Verification items for the finished model (mm, model axes). A direction names the side the tool comes from. Coordinates: 2 decimals unless noted, no trailing zeros. Loops run counter-clockwise (first coordinate to the right, second up) from the corner with the lowest first, then second, coordinate; pieces in that order, holes last.
Q1. Mould release check, pull along Z, two halves, no side actions. Record for faces 3 (the face through (1, 1, 0)), 4 (the face through (2.54, 1, -1)), 5 (the face through (1, 0.381, -2)): +Z half, -Z half, draft (parallel to the pull), parting line (faces both ways), or undercut.
Q2. Go/stop test with flat-tipped pins: P1, Ø0.5, axis at y = -1.5, z = -1.5, coming from the -X side; P2, Ø0.7, axis at x = 1.5, y = 6.5, coming from the -Z side; P3, Ø0.7, axis at x = 1, y = -0.5, coming from the +Z side. Record where each tip stops, or that it passes through.
Q3. Access from +Z, -Z, +X, -X, +Y, -Y to the whole of each face (thin tool, end or side, straight path). Record for faces 1 (the face through (0.7, 2.54, -1.3)), 2 (the face through (0, 1, -1)).
Q4. Sectioned sample at A-A (x = 1.9). Enter the section's corners in (y, z), then the cut area to 3 significant figures.
Q5. Sectioned sample at B-B (y = 7.5). Enter the section's corners in (x, z), then the cut area to 3 significant figures.
Q6. Material ranges on probe 1 along Z at (x, y) = (1, 0.25); probe 2 along Y at (x, z) = (1.35, -0.45); probe 3 along Z at (x, y) = (1.5, 3.25), recorded low to high.
Q7. Sectioned sample at C-C (z = -2.35). Enter the section's corners in (x, y), then the cut area to 3 significant figures.
```python
from build123d import *

# Parameters (mm, degrees)
SKETCH1_W             = 2.54
SKETCH1_H             = 2.54
MAIN_BODY_DEPTH       = 2.54
SKETCH3_W             = 1.778
SKETCH3_H             = 0.381
CUT_EXTRUDE1_DEPTH    = 3.54
CUT_EXTRUDE2_DEPTH    = 3.54
SKETCH2_W             = 0.64
SKETCH2_H             = 0.64
PIN_DEPTH             = 6
PIN_DEPTH_BACK        = 5.54
CHAMFER1_SIZE         = 0.508
CHAMFER1_SIZE2        = 0.1905
CHAMFER1_PART_2_SIZE  = 0.508
CHAMFER1_PART_2_SIZE2 = 0.1905
CHAMFER1_PART_3_SIZE  = 0.508
CHAMFER1_PART_3_SIZE2 = 0.1905
CHAMFER1_PART_4_SIZE  = 0.508
CHAMFER1_PART_4_SIZE2 = 0.1905
CHAMFER2_SIZE         = 0.1905
CHAMFER2_SIZE2        = 0.508


with BuildPart() as part:
    # Sketch1 → Main Body (new body)
    with BuildSketch(Plane(origin=(0, 0, 0), x_dir=(1, 0, 0), z_dir=(0, 1, 0))):
        with Locations((1.27, 1.27)):
            Rectangle(SKETCH1_W, SKETCH1_H)
    extrude(amount=MAIN_BODY_DEPTH)

    # Sketch3 → Cut-Extrude1 (cut, through all)
    with BuildSketch(Plane.ZY):
        with Locations((-1.27, 0.1905)):
            Rectangle(SKETCH3_W, SKETCH3_H)
    extrude(amount=-CUT_EXTRUDE1_DEPTH, mode=Mode.SUBTRACT)

    # Sketch4 → Cut-Extrude2 (cut, through all)
    with BuildSketch(Plane(origin=(0, 2.54, 0), x_dir=(1, 0, 0), z_dir=(0, 1, 0))):
        Polygon((0.254, 2.54), (0, 2.54), (0, 2.032), align=None)
        Polygon((2.54, 2.54), (2.286, 2.54), (2.54, 2.032), align=None)
        Polygon((0.254, 0), (0, 0.508), (0, 0), align=None)
        Polygon((2.54, 0), (2.286, 0), (2.54, 0.508), align=None)
    extrude(amount=-CUT_EXTRUDE2_DEPTH, mode=Mode.SUBTRACT)

    # Sketch2 → Pin (add, two sides)
    with BuildSketch(Plane(origin=(0, 2.54, 0), x_dir=(1, 0, 0), z_dir=(0, 1, 0))) as pin_sk:
        with Locations((1.27, 1.27)):
            Rectangle(SKETCH2_W, SKETCH2_H)
    extrude(amount=PIN_DEPTH)
    extrude(pin_sk.sketch, amount=-PIN_DEPTH_BACK)

    # Chamfer1
    chamfer1_edges = [part.edges().sort_by_distance(p)[0] for p in [
        (0.95, 8.54, -1.27),
    ]]
    chamfer1_side = [part.faces().sort_by_distance(p)[0] for p in [
        (0.95, 5.54, -1.27),
    ]]
    chamfer(chamfer1_edges, length=CHAMFER1_SIZE, length2=CHAMFER1_SIZE2, reference=chamfer1_side[0])

    # Chamfer1 part 2
    chamfer1_part_2_edges = [part.edges().sort_by_distance(p)[0] for p in [
        (1.27, 8.54, -0.95),
    ]]
    chamfer1_part_2_side = [part.faces().sort_by_distance(p)[0] for p in [
        (1.27, 5.54, -0.95),
    ]]
    chamfer(chamfer1_part_2_edges, length=CHAMFER1_PART_2_SIZE, length2=CHAMFER1_PART_2_SIZE2, reference=chamfer1_part_2_side[0])

    # Chamfer1 part 3
    chamfer1_part_3_edges = [part.edges().sort_by_distance(p)[0] for p in [
        (1.59, 8.54, -1.27),
    ]]
    chamfer1_part_3_side = [part.faces().sort_by_distance(p)[0] for p in [
        (1.59, 5.54, -1.27),
    ]]
    chamfer(chamfer1_part_3_edges, length=CHAMFER1_PART_3_SIZE, length2=CHAMFER1_PART_3_SIZE2, reference=chamfer1_part_3_side[0])

    # Chamfer1 part 4
    chamfer1_part_4_edges = [part.edges().sort_by_distance(p)[0] for p in [
        (1.27, 8.54, -1.59),
    ]]
    chamfer1_part_4_side = [part.faces().sort_by_distance(p)[0] for p in [
        (1.27, 5.54, -1.59),
    ]]
    chamfer(chamfer1_part_4_edges, length=CHAMFER1_PART_4_SIZE, length2=CHAMFER1_PART_4_SIZE2, reference=chamfer1_part_4_side[0])

    # Chamfer2
    chamfer2_edges = [part.edges().sort_by_distance(p)[0] for p in [
        (1.27, -3, -1.59),
        (0.95, -3, -1.27),
        (1.27, -3, -0.95),
        (1.59, -3, -1.27),
    ]]
    chamfer2_side = [part.faces().sort_by_distance(p)[0] for p in [
        (1.27, -3, -1.27),
    ]]
    chamfer(chamfer2_edges, length=CHAMFER2_SIZE, length2=CHAMFER2_SIZE2, reference=chamfer2_side[0])


solid = part.part
```
Geometry check:
1. face 3: +Z half
1. face 4: draft
1. face 5: undercut
2. P1: stops at x = 0.95
2. P2: stops at z = -1.59
2. P3: stops at z = -0.95
3. face 1: +Y
3. face 2: +Z, -Z, -X, +Y, -Y
4. outline: (0, -2.54) - (2.54, -2.54) - (2.54, 0) - (0, 0) - (0, -0.38) - (0.38, -0.38) - (0.38, -2.16) - (0, -2.16) - close
4. area: 5.77 mm2
5. outline: (0.95, -1.59) - (1.59, -1.59) - (1.59, -0.95) - (0.95, -0.95) - close
5. area: 0.410 mm2
6. probe 1: z = -2.54 to -2.16, -1.59 to -0.95, -0.38 to 0
6. probe 2: y = 0.38 to 2.54
6. probe 3: z = -1.59 to -0.95
7. outline: (0.16, 0) - (2.38, 0) - (2.38, 2.54) - (0.16, 2.54) - close
7. area: 5.64 mm2
